from build123d import *

# Parameters (mm, degrees)
SKETCH_R        = 75
PAD_DEPTH       = 10
SKETCH001_R     = 48.5
POCKET_DEPTH    = 5
SKETCH002_R     = 20
POCKET001_DEPTH = 5
SKETCH004_W     = 90
SKETCH004_H     = 8
POCKET002_DEPTH = 5
CHAMFER_SIZE    = 4
FILLET_R        = 3
FILLET001_R     = 3
FILLET002_R     = 3
FILLET003_R     = 3
FILLET004_R     = 3
CHAMFER001_SIZE = 1
CHAMFER002_SIZE = 1
CHAMFER003_SIZE = 1
CHAMFER004_SIZE = 1


with BuildPart() as part:
    # Sketch → Pad (new body)
    with BuildSketch(Plane.XY):
        Circle(SKETCH_R)
    extrude(amount=PAD_DEPTH)

    # Sketch001 (on Face3 of Pad) → Pocket (cut)
    with BuildSketch(Plane.XY.offset(10)):
        Circle(SKETCH001_R)
    extrude(amount=-POCKET_DEPTH, mode=Mode.SUBTRACT)

    # Sketch002 (on Face5 of Pocket) → Pocket001 (cut)
    with BuildSketch(Plane.XY.offset(5)):
        Circle(SKETCH002_R)
    extrude(amount=-POCKET001_DEPTH, mode=Mode.SUBTRACT)

    # Sketch004 (on Face6 of Pocket001) → Pocket002 (cut)
    with BuildSketch(Plane.XY.offset(5)):
        Rectangle(SKETCH004_W, SKETCH004_H)
    extrude(amount=-POCKET002_DEPTH, mode=Mode.SUBTRACT)

    # Chamfer
    chamfer_edges = [part.edges().sort_by_distance(p)[0] for p in [
        (-75, 0, 10),
    ]]
    chamfer(chamfer_edges, length=CHAMFER_SIZE)

    # Fillet
    fillet_edges = [part.edges().sort_by_distance(p)[0] for p in [
        (-48.5, 0, 10),
    ]]
    fillet(fillet_edges, radius=FILLET_R)

    # Fillet001
    fillet001_edges = [part.edges().sort_by_distance(p)[0] for p in [
        (-45, -4, 2.5),
    ]]
    fillet(fillet001_edges, radius=FILLET001_R)

    # Fillet002
    fillet002_edges = [part.edges().sort_by_distance(p)[0] for p in [
        (-45, 4, 2.5),
    ]]
    fillet(fillet002_edges, radius=FILLET002_R)

    # Fillet003
    fillet003_edges = [part.edges().sort_by_distance(p)[0] for p in [
        (45, -4, 2.5),
    ]]
    fillet(fillet003_edges, radius=FILLET003_R)

    # Fillet004
    fillet004_edges = [part.edges().sort_by_distance(p)[0] for p in [
        (45, 4, 2.5),
    ]]
    fillet(fillet004_edges, radius=FILLET004_R)

    # Chamfer001
    chamfer001_edges = [part.edges().sort_by_distance(p)[0] for p in [
        (19.595918, -4, 2.5),
    ]]
    chamfer(chamfer001_edges, length=CHAMFER001_SIZE)

    # Chamfer002
    chamfer002_edges = [part.edges().sort_by_distance(p)[0] for p in [
        (-19.595918, -4, 2.5),
    ]]
    chamfer(chamfer002_edges, length=CHAMFER002_SIZE)

    # Chamfer003
    chamfer003_edges = [part.edges().sort_by_distance(p)[0] for p in [
        (-19.595918, 4, 2.5),
    ]]
    chamfer(chamfer003_edges, length=CHAMFER003_SIZE)

    # Chamfer004
    chamfer004_edges = [part.edges().sort_by_distance(p)[0] for p in [
        (19.595918, 4, 2.5),
    ]]
    chamfer(chamfer004_edges, length=CHAMFER004_SIZE)


solid = part.part
The listing builds one solid part. Answer for the finished solid, in the listing's coordinates (mm). A direction names the side the tool comes from. Coordinates: 2 decimals unless noted, no trailing zeros. Loops run counter-clockwise (first coordinate to the right, second up) from the corner with the lowest first, then second, coordinate; pieces in that order, holes last.
1) A tool of negligible diameter and unlimited length cuts with its end or side. For faces 4 (the face through (-31, -4, 3)), 5 (the face through (16, -16, 0)), 6 (the face through (22.38, -43.028, 6.014)), from which of +Z, -Z, +X, -X, +Y, -Y can it reach the whole face along a straight path? Write none if from no direction.
2) Find section B-B on z = 3.5. Write down the section's boundary in (x, y), then the cut area to 3 significant figures.
3) Flat-ended cylindrical pins translate along their axes: pin 1 Ø1.6 at (y, z) = (0.5, 2.5) entering from -X; pin 2 Ø2.5 at (x, z) = (35, 2) entering from +Y; pin 3 Ø4 at (x, z) = (27.5, 3) entering from -Y; pin 4 Ø2 at (x, z) = (-42, 8.5) entering from +Y. Find the tip coordinate at first contact, or state that the pin passes through.
4) Find the intervals of material crossed by L1, parallel to Y at x = 0, z = 5.75; L2, parallel to X at y = 7, z = 0.5 (3 decimals); L3, parallel to Z at x = -39, y = -17.5, in increasing order.
5) Find section A-A on x = 0. Write down the section's boundary in (y, z).
6) Determine the mould class of faces 1 (the face through (-9.764, 74.362, 2.958)), 2 (the face through (-1, -21, 5)), 3 (the face through (36.5, 37.1, 10)) for opening direction Y: pulls with the +Y half, pulls with the -Y half, needs draft (parallel to the pull), parting line crosses it, or undercut.
Values:
1. face 4: +Z, -Z
1. face 5: -Z, +X, -X, +Y, -Y
1. face 6: +Z
2. outline: circle Ø150 at (0, 0); hole (-45, -1) arc R3 ccw to (-42, -4) - (-20.6, -4) - (-19.37, -4.97) arc R20 ccw to (19.37, -4.97) - (20.6, -4) - (42, -4) arc R3 ccw to (45, -1) - (45, 1) arc R3 ccw to (42, 4) - (20.6, 4) - (19.37, 4.97) arc R20 ccw to (-19.37, 4.97) - (-20.6, 4) - (-42, 4) arc R3 ccw to (-45, 1) - close
2. area: 16,000 mm2
3. pin 1: stops at x = -75
3. pin 2: stops at y = 66.98
3. pin 3: stops at y = -70.53
3. pin 4: stops at y = 60.5
4. L1: y = -75 to -48.5, 48.5 to 75
4. L2: x = -74.673 to -18.735, 18.735 to 74.673
4. L3: z = 0 to 5
5. outline: (-75, 0) - (-20, 0) - (-20, 5) - (-48.5, 5) - (-48.5, 7) arc R3 ccw to (-51.5, 10) - (-71, 10) - (-75, 6) - close; (20, 0) - (75, 0) - (75, 6) - (71, 10) - (51.5, 10) arc R3 ccw to (48.5, 7) - (48.5, 5) - (20, 5) - close
6. face 1: parting line crosses it
6. face 2: undercut
6. face 3: needs draft
